For this review, take the finished solid that the model builds, in its own axes (mm). Give positions to 0.01 mm unless a question says otherwise; leave off trailing zeros. Write each loop counter-clockwise with the first axis right and the second up, starting at its lowest first coordinate (ties: lowest second). Pieces come first, ordered by that corner, then holes.
1) For P1, Ø4, axis at y = 307.5, z = -1355.5, coming from the +X side; P2, Ø1, axis at y = 324, z = -1351, coming from the -X side; P3, Ø1.5, axis at y = 294.5, z = -1342, coming from the +X side, all flat-tipped, find the tip position at first contact; note any pin that passes through.
2) Wall thickness on line 1 along Y through (x, z) = (-113.5, -1355.5); line 2 along Y through (x, z) = (-119.5, -1354.25); line 3 along Y through (x, z) = (-118, -1347.5): over which ranges is each line inside the solid? List them lowest first.
3) Draft analysis for pull direction X (two halves, no side actions). For faces 1 (the face through (-121.25, 294.53, -1355.01)), 2 (the face through (-113.794, 309.789, -1354.146)), 3 (the face through (-106.884, 306.471, -1341.061)), state which applies: pulls with the +X half, pulls with the -X half, needs draft (parallel to the pull), parting line crosses it, or undercut.
4) We need section B-B on z = -1345.75. Give the boundary of the cut face in (x, y).
5) We need section A-A on y = 301.5. Give the boundary of the cut face in (x, z).
6) We need section C-C on x = -99. Give the boundary of the cut face in (y, z).
Autodesk Inventor part; units mm, degrees
ref_plane "Work Plane1" through (-107.0936, 321.7811, -1369.8087) normal (-0.8986472, 0.4364419, 0.044177) x (0.0175477, -0.0648608, 0.99774)
ref_plane "Work Plane2" through (-113.4024, 293.0987, -1341.5395) normal (-0.8986472, 0.4364419, 0.044177) x (0.0175477, -0.0648608, 0.99774)
ref_plane "YZ Plane" through (0, 0, 0) normal (1, 0, 0) x (0, 1, 0)
ref_plane "Work Plane1" through (-107.0936, 321.7811, -1369.8087) normal (-0.8986472, 0.4364419, 0.044177) x (0.0175477, -0.0648608, 0.99774)
sketch "Sketch2" plane through (-107.0936, 321.7811, -1369.8087) normal (-0.8986472, 0.4364419, 0.044177) x (0.0175477, -0.0648608, 0.99774)
  circle A0 centre (15, 4.5) radius 1.35
  circle A1 centre (15, -12.5) radius 1.35
  circle A2 centre (15, -29.5) radius 1.35
  line L0 (17.8, -32.6) -> (17.8, 6)
  line L1 (12.2, -30) -> (12.2, 9)
  line L2 (12.2, -34.5) -> (12.2, 9.5)
  circle A3 centre (15, 4.5) radius 1.35
  circle A4 centre (15, -12.5) radius 1.35
  circle A5 centre (15, -29.5) radius 1.35
  line L3 (12.2, 9.5) -> (31.2, 9.5)
  line L4 (12.2, -34.5) -> (31.2, -34.5)
  line L5 (31.2, 6) -> (31.2, -32.6)
  line L6 (31.2, -32.6) -> (35.7, -32.6)
  line L7 (35.7, -31.975) -> (35.7, -32.6)
  line L8 (33.7, -31.975) -> (35.7, -31.975)
  line L9 (33.7, -27.025) -> (33.7, -31.975)
  line L10 (35.7, -27.025) -> (33.7, -27.025)
  line L11 (35.7, -25.525) -> (35.7, -27.025)
  line L12 (33.2, -25.525) -> (35.7, -25.525)
  line L13 (33.2, -16.475) -> (33.2, -25.525)
  line L14 (35.7, -16.475) -> (33.2, -16.475)
  line L15 (35.7, -14.975) -> (35.7, -16.475)
  line L16 (33.7, -14.975) -> (35.7, -14.975)
  line L17 (33.7, -10.025) -> (33.7, -14.975)
  line L18 (35.7, -10.025) -> (33.7, -10.025)
  line L19 (35.7, -8.525) -> (35.7, -10.025)
  line L20 (33.2, -8.525) -> (35.7, -8.525)
  line L21 (33.2, 0.525) -> (33.2, -8.525)
  line L22 (35.7, 0.525) -> (33.2, 0.525)
  line L23 (35.7, 2.025) -> (35.7, 0.525)
  line L24 (33.7, 2.025) -> (35.7, 2.025)
  line L25 (33.7, 6) -> (33.7, 2.025)
  line L26 (33.7, 6) -> (31.2, 6)
  line L27 (31.2, 9.5) -> (31.2, -34.5)
  line L28 (28.2, 9.5) -> (28.2, -34.5)
  dimension "d1" = 2.7
  dimension "d2" = 2.7
  dimension "d3" = 2.7
  dimension "d6" = 5
  dimension "d8" = 5
  dimension "d13" = 3
extrude "Extrusion2" add sketch "Sketch2" along normal blind 3 contours L1 L2 L3 L28 L4 | L28 L3 L27 L5 L4
sketch "Sketch3" plane through (-107.0936, 321.7811, -1369.8087) normal (0.8986472, -0.4364419, -0.044177) x (-0.0175477, 0.0648608, -0.99774)
  circle A0 centre (-15, 4.5) radius 1.35
  circle A1 centre (-15, -29.5) radius 1.35
  circle A2 centre (-15, -12.5) radius 1.35
  line L0 (-31.2, -34.5) -> (-31.2, 9.5)
  line L1 (-12.2, -34.5) -> (-31.2, -34.5)
  line L2 (-12.2, 9.5) -> (-12.2, -34.5)
  line L3 (-31.2, 9.5) -> (-12.2, 9.5)
  point P0 (-1389.4632, -172.471)
sketch "Sketch4" plane through (-109.7896, 323.0904, -1369.6761) normal (-0.8986472, 0.4364419, 0.044177) x (0.0175477, -0.0648608, 0.99774)
  line L0 (12.2, -34.5) -> (31.2, -34.5)
  line L1 (31.2, 9.5) -> (28.2, 9.5)
  line L2 (28.2, 9.5) -> (28.2, -34.5)
  line L3 (28.2, -34.5) -> (31.2, -34.5)
  line L4 (31.2, -34.5) -> (31.2, 9.5)
  dimension "d16" = 3
ref_plane "Work Plane2" through (-113.4024, 293.0987, -1341.5395) normal (-0.8986472, 0.4364419, 0.044177) x (0.0175477, -0.0648608, 0.99774)
extrude "Extrusion3" add sketch "Sketch4" against normal up to surface (8.6 mm away)
sketch "Sketch5" plane through (-121.7209, 288.992, -1343.4191) normal (-0.0175477, 0.0648608, -0.99774) x (-0.8986472, 0.4364419, 0.044177)
  circle A0 centre (-2.8, 39) radius 1.35
  circle A1 centre (-2.8, 22) radius 1.35
  circle A2 centre (-2.8, 5) radius 1.35
  circle A3 centre (-2.8, 5) radius 1.35
  circle A4 centre (-2.8, 22) radius 1.35
  circle A5 centre (-2.8, 39) radius 1.35
  point P0 (-176.1642, -137.971)
  dimension "d19" = 2.7
  dimension "d20" = 2.7
  dimension "d21" = 2.7
extrude "Extrusion4" cut sketch "Sketch5" against normal through all
properties part number "Trapezium" material "Aluminum-6061"
Results list:
1. P1: stops at x = -112.51
1. P2: stops at x = -108.67
1. P3: stops at x = -112.38
2. line 1: y = 307.14 to 308.67, 311.66 to 314.02
2. line 2: y = 294.66 to 301.53
2. line 3: y = 297.07 to 303.94
3. face 1: undercut
3. face 2: undercut
3. face 3: pulls with the +X half
4. outline: (-124.46, 290.46) - (-121.76, 289.14) - (-102.51, 328.77) - (-105.21, 330.09) - close
5. outline: (-119.73, -1358.68) - (-116.4, -1358.74) - (-115.61, -1342.71) - (-109.39, -1342.82) - (-109.24, -1339.82) - (-118.8, -1339.65) - close
6. outline: (322.46, -1338.64) - (322.76, -1341.62) - (326.81, -1341.36) - (326.64, -1338.36) - close
